Verification items for the finished model (mm, model axes). A direction names the side the tool comes from. Round coordinates to 2 decimals unless told otherwise and drop trailing zeros. Write each loop counter-clockwise with the first axis right and the second up, starting at its lowest first coordinate (ties: lowest second). Pieces come first, ordered by that corner, then holes. Notation, with made-up numbers: (47, 51) - (57, 51) arc R3 cw to (57, 55) - close; hole circle Ø11 at (80.5, -25.75). An arc over 180 degrees is marked (long way). Write each question's results on one line, items separated by ' | '.
```python
from build123d import *

# Parameters (mm, degrees)
SKETCH1_W           = 66
SKETCH1_H           = 68
SKETCH1_R           = 1
SKETCH1_W_2         = 17.8
SKETCH1_H_2         = 7.6
BOSS_EXTRUDE1_DEPTH = 2
SKETCH2_W           = 16
SKETCH2_H           = 4.75
BOSS_EXTRUDE2_DEPTH = 16.3


with BuildPart() as part:
    # Sketch1 → Boss-Extrude1 (new body)
    with BuildSketch(Plane.XY.offset(30)):
        with Locations((251.940861289, 301.024014524)):
            Rectangle(SKETCH1_W, SKETCH1_H)
        with Locations((249.003592831, 330.031505481)):
            Circle(SKETCH1_R, mode=Mode.SUBTRACT)
        with Locations((255.055282531, 330.031505481)):
            Circle(SKETCH1_R, mode=Mode.SUBTRACT)
        with Locations((252.135035756, 320.823888471)):
            Rectangle(SKETCH1_W_2, SKETCH1_H_2, mode=Mode.SUBTRACT)
    extrude(amount=BOSS_EXTRUDE1_DEPTH)

    # Sketch2 → Boss-Extrude2 (add)
    with BuildSketch(Plane.XY.offset(32)):
        with Locations((236.037971242, 332.649014524)):
            Rectangle(SKETCH2_W, SKETCH2_H)
        with Locations((268, 332.649014524)):
            Rectangle(SKETCH2_W, SKETCH2_H)
    extrude(amount=BOSS_EXTRUDE2_DEPTH)


solid = part.part
```
(1) Mould release check, pull along Y, two halves, no side actions. Record for faces 6 (the flat face through (218.941, 301, 31)), 7 (the cylindrical face through (255.517, 329.144, 30.986)), 8 (the flat face through (261.035, 321, 31)), 9 (the flat face through (251, 267.024, 31)): released by +Y, released by -Y, zero draft, split by the parting line, or undercut.
Answer:
face 6: zero draft | face 7: undercut | face 8: undercut | face 9: released by -Y
(2) Go/stop test with flat-tipped pins: pin 1 Ø4 at (y, z) = (332.5, 38) entering from +X; pin 2 Ø1.8 at (x, y) = (249, 330.03) entering from -Z; pin 3 Ø5 at (y, z) = (332, 37) entering from -X; pin 4 Ø5 at (x, z) = (239, 39) entering from -Y. Record where each tip stops, or that it passes through.
Answer:
pin 1: x = 276 | pin 2: through | pin 3: x = 228.04 | pin 4: y = 330.27
(3) Set-up check for faces 1 (the flat face through (243.235, 321, 31)), 2 (the flat face through (236, 330.274, 40)), 3 (the flat face through (276, 333, 40)), 4 (the flat face through (244.038, 333, 40)), 5 (the flat face through (228.038, 333, 40)): record each of +Z, -Z, +X, -X, +Y, -Y from which the full face is reachable in a straight line by a thin tool's end or side.
Answer:
face 1: +Z, -Z | face 2: +Z, +X, -X, -Y | face 3: +Z, +X, +Y, -Y | face 4: +Z, +Y, -Y | face 5: +Z, -X, +Y, -Y
(4) Section check D-D (x = 277.5). Record the cut outline in (y, z), plus the area to 3 significant figures.
Answer:
outline: (267.02, 30) - (335.02, 30) - (335.02, 32) - (267.02, 32) - close | area: 136 mm2
(5) Section check C-C (y = 274.5). Record the cut outline in (x, z).
Answer:
outline: (218.94, 30) - (284.94, 30) - (284.94, 32) - (218.94, 32) - close
(6) Section check B-B (z = 33). Record the cut outline in (x, y), plus the area to 3 significant figures.
Answer:
outline: (228.04, 330.27) - (244.04, 330.27) - (244.04, 335.02) - (228.04, 335.02) - close; (260, 330.27) - (276, 330.27) - (276, 335.02) - (260, 335.02) - close | area: 152 mm2
(7) Thickness scan on L1, parallel to Z at x = 243.5, y = 281; L2, parallel to Y at x = 271.5, z = 32.5. Record the ranges inside material, lowest first.
Answer:
L1: 30 to 32 | L2: 330.27 to 335.02
(8) Section check A-A (x = 257). Record the cut outline in (y, z).
Answer:
outline: (267.02, 30) - (317.02, 30) - (317.02, 32) - (267.02, 32) - close; (324.62, 30) - (335.02, 30) - (335.02, 32) - (324.62, 32) - close
